```python
from build123d import *

# Parameters (mm, degrees)
BOSS_EXTRUDE1_DEPTH      = 11
BOSS_EXTRUDE1_DEPTH_BACK = 11
CUT_EXTRUDE1_REACH       = 98.151
SKETCH2_R                = 5.25
SKETCH2_R_2              = 2
BOSS_EXTRUDE2_DEPTH      = 4
FILLET1_R                = 3
FILLET2_R                = 1
SHELL1_START             = -24.5
SHELL1_DEPTH             = 35
SHELL1_START_2           = -10
SHELL1_2_DEPTH           = 20
CUT_EXTRUDE2_REACH       = 56.546
SKETCH4_W                = 25
SKETCH4_H                = 8
CHAMFER1_SIZE            = 1
DELETEFACE2_START        = -10
DELETEFACE2_DEPTH        = 20


with BuildPart() as part:
    # Sketch1 → Boss-Extrude1 (new, two sides: drawn at the far end of the back side and taken through both)
    with BuildSketch(Plane.XY.offset(-BOSS_EXTRUDE1_DEPTH_BACK)):
        with BuildLine():
            Line((-44.5, 0), (-44.5, -1))
            Line((-44.5, -1), (43.5, -1))
            ThreePointArc((43.5, -1), (44.207106781, -1.292893219), (44.5, -2))
            Line((44.5, -2), (44.5, -32))
            Line((44.5, -32), (45.5, -32))
            Line((45.5, -32), (45.5, -1))
            ThreePointArc((45.5, -1), (45.207106781, -0.292893219), (44.5, 0))
            Line((44.5, 0), (-44.5, 0))
        make_face()
    extrude(amount=BOSS_EXTRUDE1_DEPTH + BOSS_EXTRUDE1_DEPTH_BACK)

    # Sketch2 → Cut-Extrude1 (cut, up to next)
    with BuildSketch(Plane(origin=(45.5, 0, 0), x_dir=(0, 0, -1), z_dir=(1, 0, 0)), mode=Mode.PRIVATE) as cut_extrude1_sk1:
        with Locations(Location((0, -11, 0), (0, 0, 90))):
            Circle(SKETCH2_R)
    cut_extrude1_tool1 = extrude(cut_extrude1_sk1.sketch, amount=-CUT_EXTRUDE1_REACH, mode=Mode.PRIVATE) & part.part
    # Sketch2 → Cut-Extrude1 (cut, up to next)
    with BuildSketch(Plane(origin=(45.5, 0, 0), x_dir=(0, 0, -1), z_dir=(1, 0, 0)), mode=Mode.PRIVATE) as cut_extrude1_sk2:
        with Locations(Location((0, -26, 0), (0, 0, 90))):
            Circle(SKETCH2_R_2)
    cut_extrude1_tool2 = extrude(cut_extrude1_sk2.sketch, amount=-CUT_EXTRUDE1_REACH, mode=Mode.PRIVATE) & part.part
    add(cut_extrude1_tool1.solids().sort_by_distance((45.5, -11, 0))[0], mode=Mode.SUBTRACT)
    add(cut_extrude1_tool2.solids().sort_by_distance((45.5, -26, 0))[0], mode=Mode.SUBTRACT)

    # Sketch3 → Boss-Extrude2 (add)
    with BuildSketch(Plane.XZ.offset(1)):
        with BuildLine():
            Line((10.5, -6), (-24.5, -6))
            ThreePointArc((-24.5, -6), (-30.5, 0), (-24.5, 6))
            Line((-24.5, 6), (10.5, 6))
            ThreePointArc((10.5, 6), (16.5, 0), (10.5, -6))
        make_face()
    extrude(amount=BOSS_EXTRUDE2_DEPTH)

    # Fillet1
    fillet1_edges = [part.edges().sort_by_distance(p)[0] for p in [
        (16.5, -1, 0),
        (-7, -1, 6),
        (-30.5, -1, 0),
        (-7, -1, -6),
    ]]
    fillet(fillet1_edges, radius=FILLET1_R)

    # Fillet2
    fillet2_edges = [part.edges().sort_by_distance(p)[0] for p in [
        (16.5, -5, 0),
        (-7, -5, -6),
        (-30.5, -5, 0),
        (-7, -5, 6),
    ]]
    fillet(fillet2_edges, radius=FILLET2_R - 0.0001)  # a hair under: the kernel refuses the full size

    # Shell1: read off the stored shape, not the designer's step
    # Shell1 outline → Shell1 (cut)
    with BuildSketch(Plane.YZ.offset(SHELL1_START)):
        with BuildLine():
            Line((0, -9), (0, 9))
            ThreePointArc((0, 9), (-1.171572875, 6.171572875), (-4, 5))
            Line((-4, 5), (-4, -5))
            ThreePointArc((-4, -5), (-1.171572875, -6.171572875), (0, -9))
        make_face()
    extrude(amount=SHELL1_DEPTH, mode=Mode.SUBTRACT)

    # Shell1 2 outline → Shell1 2 (cut)
    with BuildSketch(Plane.XY.offset(SHELL1_START_2)):
        with BuildLine():
            ThreePointArc((43.5, 0), (44.01763809, -0.068148347), (44.5, -0.267949192))
            Line((44.5, -0.267949192), (44.5, 0))
            Line((44.5, 0), (43.5, 0))
        make_face()
    extrude(amount=SHELL1_2_DEPTH, mode=Mode.SUBTRACT)

    # Shell1 3 outline → Shell1 3 (revolve, cut)
    with BuildSketch(Plane(origin=(10.5, 0, 0), x_dir=(1, 0, 0), z_dir=(0, 0, 1))):
        with BuildLine():
            Line((9, 0), (0, 0))
            Line((0, 0), (0, -4))
            Line((0, -4), (5, -4))
            ThreePointArc((5, -4), (6.171572875, -1.171572875), (9, 0))
        make_face()
    revolve(axis=Axis((10.5, 0, 0), (0, 1, 0)), mode=Mode.SUBTRACT)

    # Shell1 4 outline → Shell1 4 (revolve, cut)
    with BuildSketch(Plane(origin=(-24.5, 0, 0), x_dir=(1, 0, 0), z_dir=(0, 0, 1))):
        with BuildLine():
            Line((9, 0), (0, 0))
            Line((0, 0), (0, -4))
            Line((0, -4), (5, -4))
            ThreePointArc((5, -4), (6.171572875, -1.171572875), (9, 0))
        make_face()
    revolve(axis=Axis((-24.5, 0, 0), (0, 1, 0)), mode=Mode.SUBTRACT)

    # Sketch4 → Cut-Extrude2 (cut, up to next)
    with BuildSketch(Plane(origin=(0, -4, 0), x_dir=(1, 0, 0), z_dir=(0, 1, 0)), mode=Mode.PRIVATE) as cut_extrude2_sk1:
        with Locations((-7, 0)):
            Rectangle(SKETCH4_W, SKETCH4_H)
    cut_extrude2_tool1 = extrude(cut_extrude2_sk1.sketch, amount=-CUT_EXTRUDE2_REACH, mode=Mode.PRIVATE) & part.part
    add(cut_extrude2_tool1.solids().sort_by_distance((-7, -4, 0))[0], mode=Mode.SUBTRACT)

    # Chamfer1
    chamfer1_edges = [part.edges().sort_by_distance(p)[0] for p in [
        (45.5, -28, 0),
    ]]
    chamfer(chamfer1_edges, length=CHAMFER1_SIZE - 0.0001)  # a hair under: the kernel refuses the full size

    # DeleteFace2: read off the stored shape, not the designer's step
    # DeleteFace2 outline → DeleteFace2 (add)
    with BuildSketch(Plane.XY.offset(DELETEFACE2_START)):
        with BuildLine():
            Line((44.5, -0.267949192), (44.5, 0))
            ThreePointArc((44.5, 0), (44.289569284, -0.022391226), (44.088562172, -0.088562172))
            ThreePointArc((44.088562172, -0.088562172), (44.299329325, -0.166677161), (44.5, -0.267949192))
        make_face()
    extrude(amount=DELETEFACE2_DEPTH)


solid = part.part
```
Geometry: final body of the model. Coordinates: model frame, mm. A direction names the side the tool comes from. Round coordinates to 2 decimals unless told otherwise and drop trailing zeros. Order: outer loops, then holes, each group sorted by start corner. A loop starts at its lowest first (then second) coordinate and runs counter-clockwise, first axis right, second up. Notation, with made-up numbers: (-39.5, 6.25) -> (9.5, 6.25) arc R22 cw to (9.5, 16.25) -> close; hole circle Ø1 at (72, -1.75). An arc over 180 degrees is marked (long way). Use one line per item in the form item = value. Start each with the question number.
1. Pin query (flat end, axial travel): pin 1 Ø8 at (x, y) = (15, -6) entering from +Z; pin 2 Ø4 at (y, z) = (-17, -0.5) entering from -X; pin 3 Ø11 at (x, z) = (-19, 4.5) entering from -Y; pin 4 Ø6.5 at (y, z) = (-11, 0) entering from -X. Return the tip coordinate at first contact, or that it passes through.
2. Reachability of faces 1 (the face through (-6.7, -5, -4.4)), 2 (the face through (-7.3, -4, -4.4)), 3 (the face through (45.5, -17, 0)), 4 (the face through (9, -1, -10)), 5 (the face through (-6.75, -1.86, 6.9)) from +Z, -Z, +X, -X, +Y, -Y: full face, straight path, thin tool, end or side. Return the list, or none.
3. Cut plane D-D (x = 26.5). Return the cut outline in (y, z), then the cut area to 3 significant figures.
4. Cut plane B-B (z = 0). Count the separate pieces of the cut face and the enclosed holes in it, then the cut area to 3 significant figures.
5. Line query: probe 1 along X at (y, z) = (-3.5, 4); probe 2 along Z at (x, y) = (44.8, -11); probe 3 along X at (y, z) = (-5.5, 5.75). Output: solid intervals per line, ascending.
6. Draft query along Y for faces 6 (the face through (-7.245, -1.141, 6.203)), 7 (the face through (45, -6, 1.6)), 8 (the face through (-7.25, -1.86, -6.9)). Return one class per face: pulls with the +Y half, pulls with the -Y half, needs draft (parallel to the pull), parting line crosses it, or undercut.
7. Cut plane C-C (y = -11). Return the cut outline in (x, z).
Solution:
q1.pin_1 = 5.91
q1.pin_2 = 44.5
q1.pin_3 = -5
q1.pin_4 = through
q2.face_1 = +Z, -Z, -X, -Y
q2.face_2 = +Y
q2.face_3 = +Z, -Z, +X, +Y, -Y
q2.face_4 = -Y
q2.face_5 = +Z, -X, -Y
q3.outline = (-1, -11) -> (0, -11) -> (0, 11) -> (-1, 11) -> close
q3.area = 22.0 mm^2
q4.separate_pieces = 4
q4.enclosed_holes = 0
q4.area = 85.0 mm^2
q5.probe_1 = -29.03 to -27.55, 13.55 to 15.03, 44.5 to 45.5
q5.probe_2 = -11 to -5.25, 5.25 to 11
q5.probe_3 = 44.5 to 45.5
q6.face_6 = pulls with the +Y half
q6.face_7 = undercut
q6.face_8 = pulls with the -Y half
q7.outline = (44.5, -11) -> (45.5, -11) -> (45.5, -5.25) -> (44.5, -5.25) -> close; (44.5, 5.25) -> (45.5, 5.25) -> (45.5, 11) -> (44.5, 11) -> close
